Design review of the part built by this model. Coordinates are the model's own, in mm. Coordinates: 2 decimals unless noted, no trailing zeros. Write each loop counter-clockwise with the first axis right and the second up, starting at its lowest first coordinate (ties: lowest second). Pieces come first, ordered by that corner, then holes.
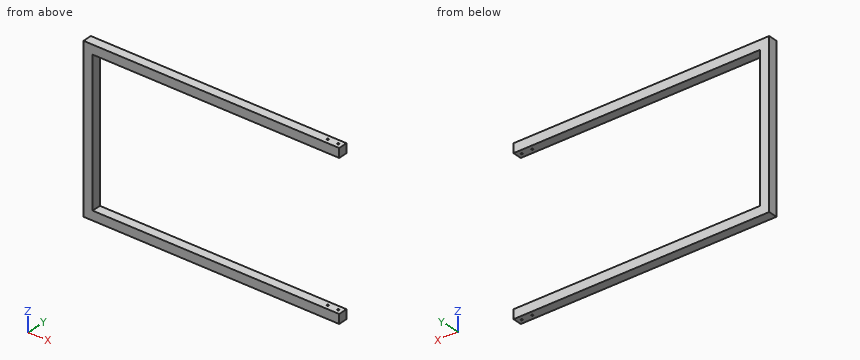
```python
from build123d import *

# Parameters (mm, degrees)
SKETCH_1_W               = 1980
SKETCH_1_H               = 530
SKETCH_1_W_2             = 1920
SKETCH_1_H_2             = 470
EXTRUDE_1_DEPTH          = 30
SKETCH_2_W               = 68
SKETCH_2_H               = 30
EXTRUDE_2_DEPTH          = 68
SKETCH_3_R               = 23.5
CUT_EXTRUDE_1_DEPTH      = 1125.999555555
SKETCH_4_W               = 31
SKETCH_4_H               = 470
EXTRUDE_3_DEPTH          = 30
SKETCH_5_R               = 3
CUT_EXTRUDE_2_DEPTH      = 1030.528532873
SKETCH_6_R               = 3
CUT_EXTRUDE_3_DEPTH      = 1030.528532873
SKETCH_7_W               = 1260.245327066
SKETCH_7_H               = 30
CUT_EXTRUDE_4_DEPTH      = 1125.999555555
CUT_EXTRUDE_5_DEPTH      = 1124.343224487
CUT_EXTRUDE_5_DEPTH_BACK = 1124.343224487
SKETCH_8_R               = 3
SKETCH_9_R               = 3
CUT_EXTRUDE_6_DEPTH      = 1124.343224487


with BuildPart() as part:
    # 草图1 → 凸台-拉伸1 (new body)
    with BuildSketch(Plane(origin=(0, 0, 0), x_dir=(1, 0, 0), z_dir=(0, 1, 0))):
        Rectangle(SKETCH_1_W, SKETCH_1_H)
        Rectangle(SKETCH_1_W_2, SKETCH_1_H_2, mode=Mode.SUBTRACT)
    extrude(amount=EXTRUDE_1_DEPTH)

    # 草图2 → 凸台-拉伸2 (add)
    with BuildSketch(Plane.XZ):
        with Locations((0, 250)):
            Rectangle(SKETCH_2_W, SKETCH_2_H)
        with Locations((0, -250)):
            Rectangle(SKETCH_2_W, SKETCH_2_H)
    extrude(amount=EXTRUDE_2_DEPTH)

    # 草图3 → 切除-拉伸1 (cut, through all)
    with BuildSketch(Plane.XY.offset(265)):
        with Locations((0, -30)):
            Circle(SKETCH_3_R)
    extrude(amount=-CUT_EXTRUDE_1_DEPTH, mode=Mode.SUBTRACT)

    # 草图4 → 凸台-拉伸3 (add)
    with BuildSketch(Plane(origin=(0, 30, 0), x_dir=(1, 0, 0), z_dir=(0, 1, 0))):
        with Locations((764.5, 0)):
            Rectangle(SKETCH_4_W, SKETCH_4_H)
    extrude(amount=-EXTRUDE_3_DEPTH)

    # 草图5 → 切除-拉伸2 (cut, through all)
    with BuildSketch(Plane(origin=(0, 30, 0), x_dir=(1, 0, 0), z_dir=(0, 1, 0))):
        with Locations(Location((759, 180, 0), (0, 0, 270))):
            Circle(SKETCH_5_R)
        with Locations(Location((774.5, 180, 0), (0, 0, 270))):
            Circle(SKETCH_5_R)
        with Locations(Location((759, -180, 0), (0, 0, 270))):
            Circle(SKETCH_5_R)
        with Locations(Location((774.5, -180, 0), (0, 0, 270))):
            Circle(SKETCH_5_R)
    extrude(amount=-CUT_EXTRUDE_2_DEPTH, mode=Mode.SUBTRACT)

    # 草图6 → 切除-拉伸3 (cut, symmetric)
    with BuildSketch(Plane(origin=(0, 30, 0), x_dir=(1, 0, 0), z_dir=(0, 1, 0))):
        with Locations(Location((840, -250, 0), (0, 0, 270))):
            Circle(SKETCH_6_R)
    cut_extrude_3 = extrude(amount=CUT_EXTRUDE_3_DEPTH, both=True, mode=Mode.SUBTRACT)

    # 镜向1: 切除-拉伸3 across plane
    add(cut_extrude_3.mirror(Plane.XY), mode=Mode.SUBTRACT)

    # 草图7 → 切除-拉伸4 (cut, through all)
    with BuildSketch(Plane.XY.offset(265)):
        with Locations((480.122663533, 15)):
            Rectangle(SKETCH_7_W, SKETCH_7_H)
    extrude(amount=-CUT_EXTRUDE_4_DEPTH, mode=Mode.SUBTRACT)


with BuildPart() as body_2:
    # of the pieces the cut leaves, the one that is kept (cut_extrude_4_keep)
    add(part.part.solids().sort_by_distance((-990, 0, -265))[0])

    # 草图8 → 切除-拉伸5 (cut, two sides: drawn at the far end of the back side and taken through both)
    with BuildSketch(Plane.XY.offset(265).offset(-CUT_EXTRUDE_5_DEPTH_BACK)):
        with Locations(Location((-200, 15, 0), (0, 0, 180))):
            Circle(SKETCH_8_R)
    extrude(amount=CUT_EXTRUDE_5_DEPTH + CUT_EXTRUDE_5_DEPTH_BACK, mode=Mode.SUBTRACT)

    # 草图9 → 切除-拉伸6 (cut, through all)
    with BuildSketch(Plane.XY.offset(265)):
        with Locations((-165, 15)):
            Circle(SKETCH_9_R)
    extrude(amount=-CUT_EXTRUDE_6_DEPTH, mode=Mode.SUBTRACT)


solid = body_2.part
```
(1) Wall thickness on line 1 (Z direction, x = -718.5, y = 17.25); line 2 (Y direction, x = -165, z = -242); line 3 (X direction, y = 19.5, z = -152.5): over which ranges is each line inside the solid? List them lowest first.
(2) Insertion check: pin 1 Ø1.5 at (y, z) = (20.5, 137) entering from +X; pin 2 Ø3.5 at (x, y) = (-200, 15) entering from -Z. Each pin has a flat end and moves straight along its axis. Give the tip position at first contact, or say it passes through.
(3) Consider section C-C (z = 159.5). Give the boundary of the cut face in (x, y).
(4) Consider section B-B (y = 5). Give the boundary of the cut face in (x, z), plus the area to 3 significant figures.
(5) Consider section A-A (x = -879.5). Give the boundary of the cut face in (y, z), plus the area to 3 significant figures.
Results:
1. line 1: z = -265 to -235, 235 to 265
1. line 2: y = 0 to 12, 18 to 30
1. line 3: x = -990 to -960
2. pin 1: stops at x = -960
2. pin 2: passes through
3. outline: (-990, 0) - (-960, 0) - (-960, 30) - (-990, 30) - close
4. outline: (-990, -265) - (-150, -265) - (-150, -235) - (-960, -235) - (-960, 235) - (-150, 235) - (-150, 265) - (-990, 265) - close
4. area: 64,500 mm2
5. outline: (0, -265) - (30, -265) - (30, -235) - (0, -235) - close; (0, 235) - (30, 235) - (30, 265) - (0, 265) - close
5. area: 1,800 mm2
